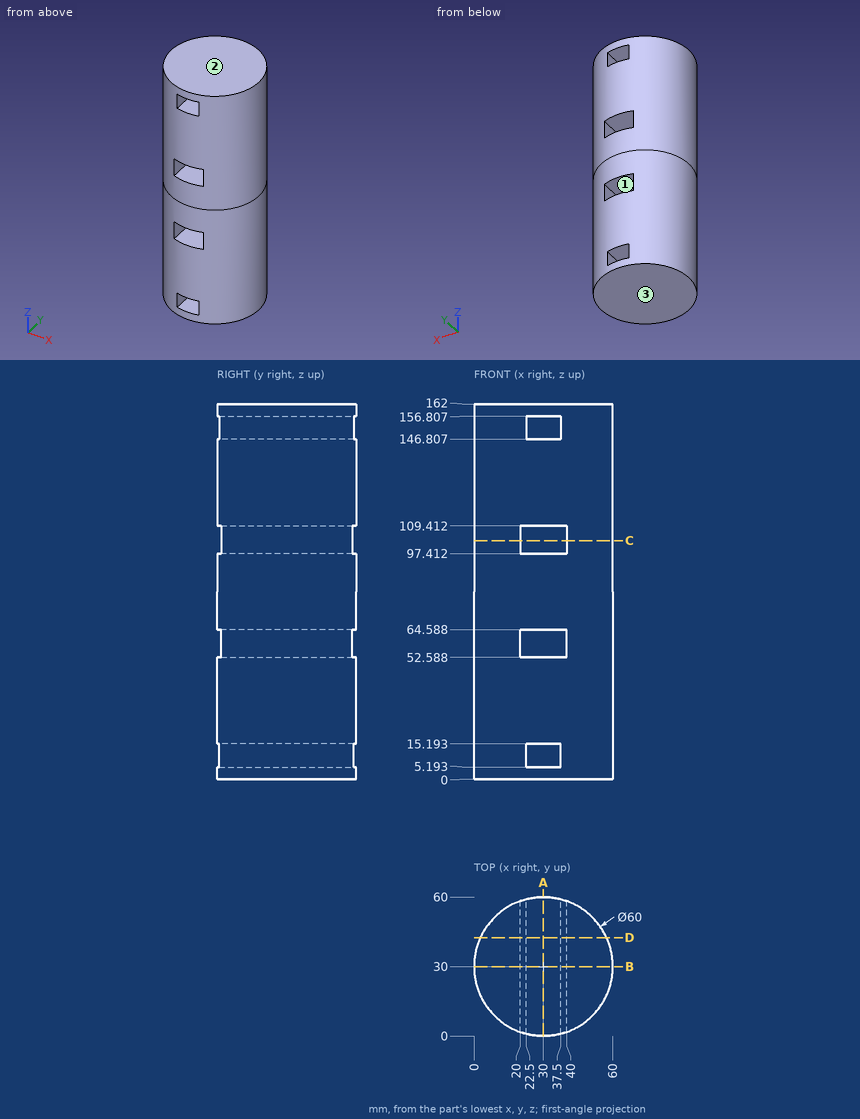
Study the drawing (mm; zero at the part's minimum x, y, z) and answer. Give positions to 0.01 mm unless a question says otherwise; leave off trailing zeros. Order: outer loops, then holes, each group sorted by start corner. A loop starts at its lowest first (then second) coordinate and runs counter-clockwise, first axis right, second up. Notation, with made-up numbers: M 38,-14.75 L 57,-14.75 A14 cw 57,5.25 Z; hole C -25.75,9 d2. An arc over 180 degrees is marked long. Put each result on its own line as item: value. Start each with the question number.
Item 1: The part is cut by section D-D, the plane y = 42.5. Determine the outline of the cut face in (x, z).
Item 2: For a pull along Z with two mould halves and no side action, classify the marked faces 1, 2 and 3 as +Z half, -Z half, draft (parallel to the pull), parting line (faces both ways), or undercut.
Item 3: Flat-ended cylindrical pins translate along their axes: P1, Ø6, axis at y = 16, z = 104, coming from the -X side; P2, Ø3, axis at x = 43.5, z = 89, coming from the -Y side (1 decimal); P3, Ø1, axis at y = 8.5, z = 127, coming from the -X side (1 decimal). Find the tip coordinate at first contact, or state that the pin passes through.
Item 4: Find the intervals of material crossed by line 1 along Z through (x, y) = (26.5, 22.5); line 2 along Z through (x, y) = (22, 37); line 3 along X through (y, z) = (29.5, 154) (1 decimal), in increasing order.
Item 5: The part is cut by section C-C, the plane z = 103. Determine the outline of the cut face in (x, y) (1 decimal), and give its area (3 significant figures).
Item 6: The part is cut by section A-A, the plane x = 30. Determine the outline of the cut face in (y, z).
Item 7: The part is cut by section B-B, the plane y = 30. Determine the outline of the cut face in (x, z).
Answer key:
1. outline: M 2.73,0 L 57.27,0 L 57.27,162 L 2.73,162 Z; hole M 20,52.59 L 40,52.59 L 40,64.59 L 20,64.59 Z; hole M 20,97.41 L 40,97.41 L 40,109.41 L 20,109.41 Z; hole M 22.5,5.19 L 37.5,5.19 L 37.5,15.19 L 22.5,15.19 Z; hole M 22.5,146.81 L 37.5,146.81 L 37.5,156.81 L 22.5,156.81 Z
2. face 1: undercut
2. face 2: +Z half
2. face 3: -Z half
3. P1: stops at x = 2.09
3. P2: stops at y = 2.5
3. P3: stops at x = 8.6
4. line 1: z = 0 to 5.19, 15.19 to 52.59, 64.59 to 97.41, 109.41 to 146.81, 156.81 to 162
4. line 2: z = 0 to 52.59, 64.59 to 97.41, 109.41 to 162
4. line 3: x = 0 to 22.5, 37.5 to 60
5. outline: M 20,1.7 L 20,58.3 A30 ccw Z; M 40,1.7 A30 ccw 40,58.3 Z
5. area: 1,650 mm²
6. outline: M 0,0 L 60,0 L 60,5.19 L 0,5.19 Z; M 0,15.19 L 60,15.19 L 60,52.59 L 0,52.59 Z; M 0,64.59 L 60,64.59 L 60,97.41 L 0,97.41 Z; M 0,109.41 L 60,109.41 L 60,146.81 L 0,146.81 Z; M 0,156.81 L 60,156.81 L 60,162 L 0,162 Z
7. outline: M 0,0 L 60,0 L 60,162 L 0,162 Z; hole M 20,52.59 L 40,52.59 L 40,64.59 L 20,64.59 Z; hole M 20,97.41 L 40,97.41 L 40,109.41 L 20,109.41 Z; hole M 22.5,5.19 L 37.5,5.19 L 37.5,15.19 L 22.5,15.19 Z; hole M 22.5,146.81 L 37.5,146.81 L 37.5,156.81 L 22.5,156.81 Z
